from build123d import *

# Parameters (mm, degrees)
SKETCH_1_R      = 2.5
EXTRUDE_1_DEPTH = 430


with BuildPart() as part:
    # 草图1 → 凸台-拉伸1 (new body)
    with BuildSketch(Plane.XY):
        with BuildLine():
            Line((14.8, 34.821428571), (18.9, 34.821428571))
            Line((18.9, 34.821428571), (20.2, 33.021428571))
            Line((20.2, 33.021428571), (17.8, 33.021428571))
            Line((17.8, 33.021428571), (17.8, 31.311378065))
            Line((17.8, 31.311378065), (20.389949494, 28.721428571))
            Line((20.389949494, 28.721428571), (26.210050506, 28.721428571))
            Line((26.210050506, 28.721428571), (28.8, 31.311378065))
            Line((28.8, 31.311378065), (28.8, 33.021428571))
            Line((28.8, 33.021428571), (26.4, 33.021428571))
            Line((26.4, 33.021428571), (27.7, 34.821428571))
            Line((27.7, 34.821428571), (38.9, 34.821428571))
            Line((38.9, 34.821428571), (40.2, 33.021428571))
            Line((40.2, 33.021428571), (37.8, 33.021428571))
            Line((37.8, 33.021428571), (37.8, 31.311378065))
            Line((37.8, 31.311378065), (40.389949494, 28.721428571))
            Line((40.389949494, 28.721428571), (46.210050506, 28.721428571))
            Line((46.210050506, 28.721428571), (48.8, 31.311378065))
            Line((48.8, 31.311378065), (48.8, 33.021428571))
            Line((48.8, 33.021428571), (46.4, 33.021428571))
            Line((46.4, 33.021428571), (47.7, 34.821428571))
            Line((47.7, 34.821428571), (51.8, 34.821428571))
            ThreePointArc((51.8, 34.821428571), (52.860660172, 34.382088743), (53.3, 33.321428571))
            Line((53.3, 33.321428571), (53.3, 29.221428571))
            Line((53.3, 29.221428571), (51.5, 27.921428571))
            Line((51.5, 27.921428571), (51.5, 30.321428571))
            Line((51.5, 30.321428571), (49.789949494, 30.321428571))
            Line((49.789949494, 30.321428571), (47.2, 27.731479078))
            Line((47.2, 27.731479078), (47.2, 21.911378065))
            Line((47.2, 21.911378065), (49.789949494, 19.321428571))
            Line((49.789949494, 19.321428571), (51.5, 19.321428571))
            Line((51.5, 19.321428571), (51.5, 21.721428571))
            Line((51.5, 21.721428571), (53.3, 20.421428571))
            Line((53.3, 20.421428571), (53.3, 16.321428571))
            ThreePointArc((53.3, 16.321428571), (52.860660172, 15.2607684), (51.8, 14.821428571))
            Line((51.8, 14.821428571), (47.7, 14.821428571))
            Line((47.7, 14.821428571), (46.4, 16.621428571))
            Line((46.4, 16.621428571), (48.8, 16.621428571))
            Line((48.8, 16.621428571), (48.8, 18.331479078))
            Line((48.8, 18.331479078), (46.210050506, 20.921428571))
            Line((46.210050506, 20.921428571), (40.389949494, 20.921428571))
            Line((40.389949494, 20.921428571), (37.8, 18.331479078))
            Line((37.8, 18.331479078), (37.8, 16.621428571))
            Line((37.8, 16.621428571), (40.2, 16.621428571))
            Line((40.2, 16.621428571), (38.9, 14.821428571))
            Line((38.9, 14.821428571), (27.7, 14.821428571))
            Line((27.7, 14.821428571), (26.4, 16.621428571))
            Line((26.4, 16.621428571), (28.8, 16.621428571))
            Line((28.8, 16.621428571), (28.8, 18.331479078))
            Line((28.8, 18.331479078), (26.210050506, 20.921428571))
            Line((26.210050506, 20.921428571), (20.389949494, 20.921428571))
            Line((20.389949494, 20.921428571), (17.8, 18.331479078))
            Line((17.8, 18.331479078), (17.8, 16.621428571))
            Line((17.8, 16.621428571), (20.2, 16.621428571))
            Line((20.2, 16.621428571), (18.9, 14.821428571))
            Line((18.9, 14.821428571), (14.8, 14.821428571))
            ThreePointArc((14.8, 14.821428571), (13.739339828, 15.2607684), (13.3, 16.321428571))
            Line((13.3, 16.321428571), (13.3, 20.421428571))
            Line((13.3, 20.421428571), (15.1, 21.721428571))
            Line((15.1, 21.721428571), (15.1, 19.321428571))
            Line((15.1, 19.321428571), (16.810050506, 19.321428571))
            Line((16.810050506, 19.321428571), (19.4, 21.911378065))
            Line((19.4, 21.911378065), (19.4, 27.731479078))
            Line((19.4, 27.731479078), (16.810050506, 30.321428571))
            Line((16.810050506, 30.321428571), (15.1, 30.321428571))
            Line((15.1, 30.321428571), (15.1, 27.921428571))
            Line((15.1, 27.921428571), (13.3, 29.221428571))
            Line((13.3, 29.221428571), (13.3, 33.321428571))
            ThreePointArc((13.3, 33.321428571), (13.739339828, 34.382088743), (14.8, 34.821428571))
        make_face()
        with Locations((23.3, 24.821428571)):
            Circle(SKETCH_1_R, mode=Mode.SUBTRACT)
        with Locations((43.3, 24.821428571)):
            Circle(SKETCH_1_R, mode=Mode.SUBTRACT)
        Polygon((27.2, 27.731479078), (29.789949494, 30.321428571), (29.789949494, 33.021428571), (36.810050506, 33.021428571), (36.810050506, 30.321428571), (39.4, 27.731479078), (39.4, 21.911378065), (36.810050506, 19.321428571), (36.810050506, 16.621428571), (29.789949494, 16.621428571), (29.789949494, 19.321428571), (27.2, 21.911378065), align=None, mode=Mode.SUBTRACT)
    extrude(amount=EXTRUDE_1_DEPTH)


solid = part.part
Here's how the part is built. I have some questions about the finished solid (model axes, mm). A direction names the side the tool comes from. Round coordinates to 2 decimals unless told otherwise and drop trailing zeros. One line per question, with ' | ' between items.
1) I need wall thicknesses on line 1 (X direction, y = 18, z = 257.5); line 2 (X direction, y = 27.5, z = 131); line 3 (Y direction, x = 23.3, z = 311.5). Which ranges of each line are inside material? Lowest first, please.
Checked values:
line 1: x = 13.3 to 17.8, 28.8 to 29.79, 36.81 to 37.8, 48.8 to 53.3 | line 2: x = 19.4 to 27.2, 39.4 to 47.2 | line 3: y = 20.92 to 22.32, 27.32 to 28.72
2) Imagine slicing it at A-A, the plane z = 229. Count the separate pieces of the cut face and the enclosed holes in it, plus the area to 3 significant figures.
Checked values:
separate pieces: 1 | enclosed holes: 3 | area: 276 mm²
3) I'm going to push flat-ended pins straight in: pin 1 Ø1.2 at (y, z) = (28.5, 145) entering from -X; pin 2 Ø1.7 at (x, z) = (22, 175) entering from -Y; pin 3 Ø3 at (y, z) = (25.5, 175.5) entering from -X; pin 4 Ø1.5 at (x, y) = (46.5, 18) entering from -Z. Where does each tip first touch, or does it pass through?
Checked values:
pin 1: stops at x = 13.47 | pin 2: stops at y = 20.92 | pin 3: stops at x = 19.4 | pin 4: passes through
4) On a 3-axis mill with a long thin cutter (end or side, diameter ignored), from which of +Z, -Z, +X, -X, +Y, -Y can I reach the whole of each face in a straight line? I mean faces 1 (the flat face through (33, 14.821, 212)), 2 (the flat face through (33, 16.621, 212)). Say none if no direction works.
Checked values:
face 1: +Z, -Z, +X, -X, -Y | face 2: +Z, -Z
